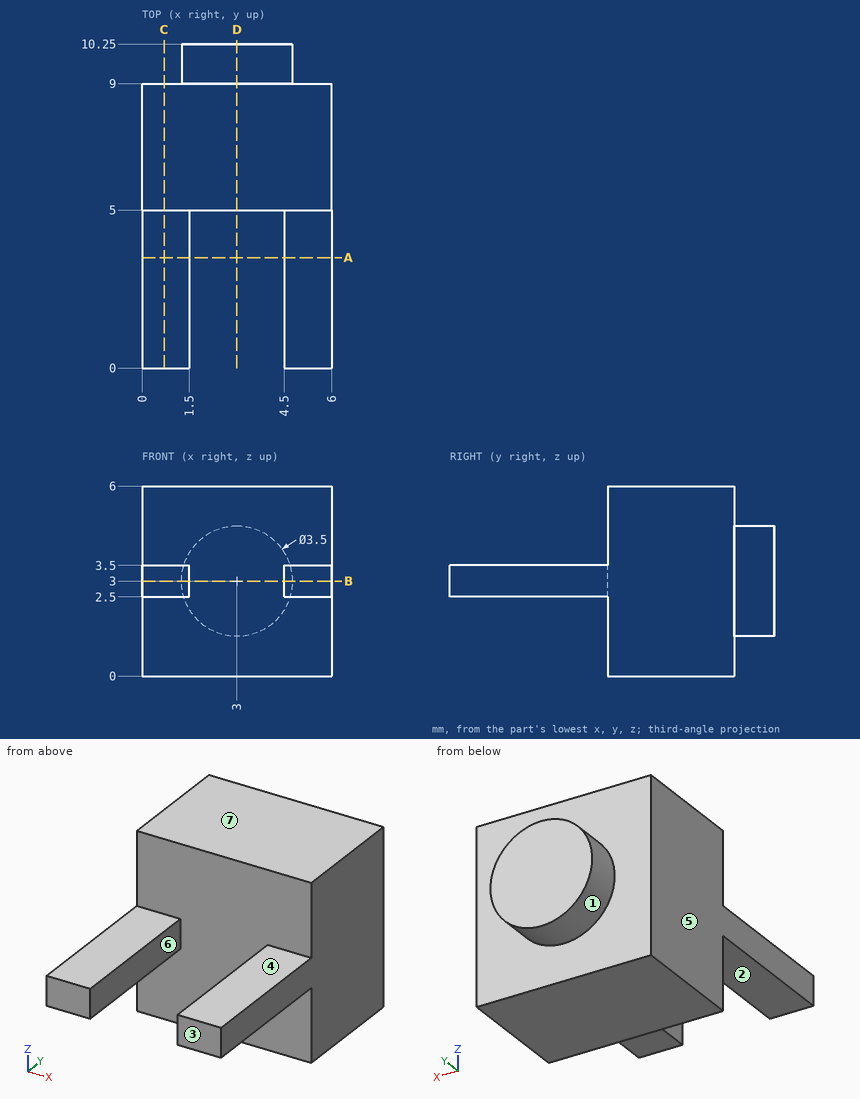
For this review, use the dimensioned drawing (mm, ordinates from the lowest corner) and the shaded views. A direction names the side the tool comes from. Give positions to 0.01 mm unless a question says otherwise; leave off trailing zeros. Order: outer loops, then holes, each group sorted by start corner. A loop starts at its lowest first (then second) coordinate and runs counter-clockwise, first axis right, second up. Notation, with made-up numbers: (30.25, 6.5) -> (81.25, 6.5) arc R33 cw to (81.25, 41.5) -> close; hole circle Ø7 at (6, 23). An arc over 180 degrees is marked (long way). Write item = value, one per line. Start each with the question number.
(1) For L1, parallel to X at y = 3.5, z = 3.3; L2, parallel to Y at x = 0.5, z = 1.2; L3, parallel to X at y = 9.5, z = 3.9, list the stretches that pass through material, from the lowest coordinate up. Write a range as from..to.
(2) Take a section at B-B (z = 3). Write out the cut boundary in (x, y), plus the area to 3 significant figures.
(3) Draft analysis for pull direction X (two halves, no side actions). For the marked faces 5, 6 and 7, state which applies: +X half, -X half, draft (parallel to the pull), parting line (faces both ways), or undercut.
(4) Take a section at D-D (x = 3). Write out the cut boundary in (y, z).
(5) For pin 1 Ø1.6 at (x, y) = (5, 1.5) entering from -Z; pin 2 Ø1 at (x, z) = (2, 4.5) entering from -Y; pin 3 Ø1.2 at (x, y) = (0.5, 1.5) entering from +Z, all flat-tipped, find the tip position at first contact; note any pin that passes through.
(6) Tool access review of the marked faces 1, 2, 3 and 4: name each direction out of +Z, -Z, +X, -X, +Y, -Y from which nothing blocks a thin tool from reaching the whole face with its end or side.
(7) Take a section at A-A (y = 3.5). Write out the cut boundary in (x, z), plus the area to 3 significant figures.
(8) Take a section at C-C (x = 0.7). Write out the cut boundary in (y, z), plus the area to 3 significant figures.
Returned:
q1.L1 = 0..1.5, 4.5..6
q1.L2 = 5..9
q1.L3 = 1.5..4.5
q2.outline = (0, 0) -> (1.5, 0) -> (1.5, 5) -> (4.5, 5) -> (4.5, 0) -> (6, 0) -> (6, 9) -> (4.75, 9) -> (4.75, 10.25) -> (1.25, 10.25) -> (1.25, 9) -> (0, 9) -> close
q2.area = 43.4 mm²
q3.face_5 = -X half
q3.face_6 = undercut
q3.face_7 = draft
q4.outline = (5, 0) -> (9, 0) -> (9, 1.25) -> (10.25, 1.25) -> (10.25, 4.75) -> (9, 4.75) -> (9, 6) -> (5, 6) -> close
q5.pin_1 = 2.5
q5.pin_2 = 5
q5.pin_3 = 3.5
q6.face_1 = +Y
q6.face_2 = -Z, +X, -X, -Y
q6.face_3 = +Z, -Z, +X, -X, -Y
q6.face_4 = +Z, +X, -X, -Y
q7.outline = (0, 2.5) -> (1.5, 2.5) -> (1.5, 3.5) -> (0, 3.5) -> close; (4.5, 2.5) -> (6, 2.5) -> (6, 3.5) -> (4.5, 3.5) -> close
q7.area = 3.00 mm²
q8.outline = (0, 2.5) -> (5, 2.5) -> (5, 0) -> (9, 0) -> (9, 6) -> (5, 6) -> (5, 3.5) -> (0, 3.5) -> close
q8.area = 29.0 mm²
